```python
from build123d import *

# Parameters (mm, degrees)
EXTRUDE_1_DEPTH = 10
FILLET_1_R      = 0.5


with BuildPart() as part:
    # 草图1 → 凸台-拉伸1 (new body)
    with BuildSketch(Plane.XY):
        with BuildLine():
            Line((4.1, 0), (0, 0))
            Line((0, 0), (0, -10))
            Line((0, -10), (4.584668807, -10))
            ThreePointArc((4.584668807, -10), (3.919335757, -6.923531768), (6.75, -8.3))
            ThreePointArc((6.75, -8.3), (6.376468232, -9.380664243), (5.415331193, -10))
            Line((5.415331193, -10), (10, -10))
            Line((10, -10), (10, 0))
            Line((10, 0), (5.9, 0))
            ThreePointArc((5.9, 0), (6.341640786, -0.529179607), (6.5, -1.2))
            ThreePointArc((6.5, -1.2), (4.329179607, -2.541640786), (4.1, 0))
        make_face()
    extrude(amount=EXTRUDE_1_DEPTH)

    # 圆角1
    fillet_1_edges = [part.edges().sort_by_distance(p)[0] for p in [
        (4.584668807, -10, 5),
        (4.1, 0, 5),
        (5.9, 0, 5),
        (5.415331193, -10, 5),
    ]]
    fillet(fillet_1_edges, radius=FILLET_1_R)


solid = part.part
```
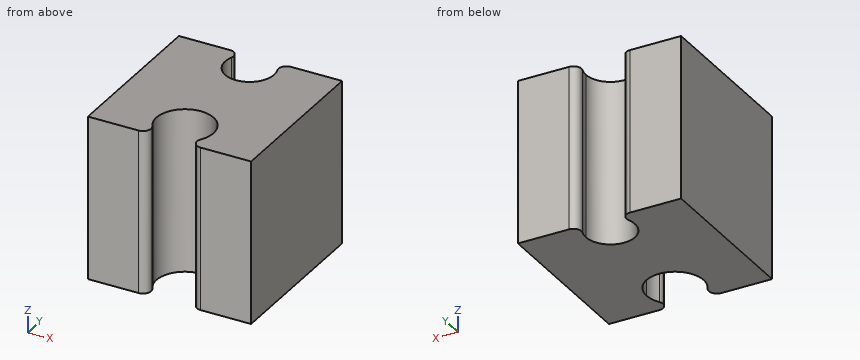
Check sheet for the modelled part. Datum: model origin and axes. Units: mm. Give positions to 0.01 mm unless a question says otherwise; leave off trailing zeros. Order: outer loops, then holes, each group sorted by start corner. A loop starts at its lowest first (then second) coordinate and runs counter-clockwise, first axis right, second up. Notation, with made-up numbers: (67.25, 1) -> (92.25, 1) arc R24 ccw to (92.25, 30) -> close; hole circle Ø2 at (-17.75, -1.5). An arc over 180 degrees is marked (long way). Return JSON: item names as keys, results as strings.
1. Cross-section at B-B, the plane x = 5. Record the cut outline in (y, z), plus the area to 3 significant figures.
From the geometry:
{"outline": "(-6.55, 0) -> (-2.7, 0) -> (-2.7, 10) -> (-6.55, 10) -> close", "area": "38.5 mm^2"}
2. Cross-section at A-A, the plane y = -9.5. Record the cut outline in (x, z), plus the area to 3 significant figures.
From the geometry:
{"outline": "(0, 0) -> (3.6, 0) -> (3.6, 10) -> (0, 10) -> close; (6.4, 0) -> (10, 0) -> (10, 10) -> (6.4, 10) -> close", "area": "71.9 mm^2"}
3. Cross-section at D-D, the plane y = -2.25. Record the cut outline in (x, z), plus the area to 3 significant figures.
From the geometry:
{"outline": "(0, 0) -> (3.93, 0) -> (3.93, 10) -> (0, 10) -> close; (6.07, 0) -> (10, 0) -> (10, 10) -> (6.07, 10) -> close", "area": "78.6 mm^2"}
4. Material ranges on probe 1 along X at (y, z) = (-1.2, 6.5); probe 2 along X at (y, z) = (-8.3, 6.5); probe 3 along Y at (x, z) = (5, 4.25), recorded low to high. Write a range as [from, to].
From the geometry:
{"probe 1": "[0, 3.5], [6.5, 10]", "probe 2": "[0, 3.25], [6.75, 10]", "probe 3": "[-6.55, -2.7]"}
